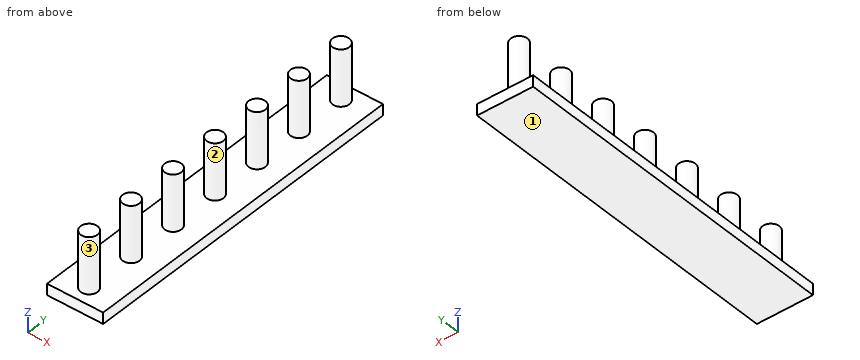
from build123d import *

# Parameters (mm, degrees)
SKETCH_1_W      = 100
SKETCH_1_H      = 600
EXTRUDE_1_DEPTH = 20
SKETCH_2_R      = 15
EXTRUDE_2_DEPTH = 100


with BuildPart() as part:
    # 草图1 → 凸台-拉伸1 (new body)
    with BuildSketch(Plane.XY):
        Rectangle(SKETCH_1_W, SKETCH_1_H)
    extrude(amount=EXTRUDE_1_DEPTH)

    # 草图2 → 凸台-拉伸2 (add)
    with BuildSketch(Plane.XY.offset(20)):
        Circle(SKETCH_2_R)
        with Locations((0, 90)):
            Circle(SKETCH_2_R)
        with Locations((0, 180)):
            Circle(SKETCH_2_R)
        with Locations((0, 270)):
            Circle(SKETCH_2_R)
        with Locations((0, -90)):
            Circle(SKETCH_2_R)
        with Locations((0, -180)):
            Circle(SKETCH_2_R)
        with Locations((0, -270)):
            Circle(SKETCH_2_R)
    extrude(amount=EXTRUDE_2_DEPTH)


solid = part.part
The listing builds one solid part. Answer for the finished solid, in the listing's coordinates (mm). Face numbers are marked on the shaded views. Round coordinates to 2 decimals unless told otherwise and drop trailing zeros. Loops run counter-clockwise (first coordinate to the right, second up) from the corner with the lowest first, then second, coordinate; pieces in that order, holes last. Notation, with made-up numbers: M 24,-5 L 75,-5 A32 cw 75,26 Z; hole C 34.25,61.5 d11. An arc over 180 degrees is marked long. Return JSON: item names as keys, results as strings.
Q1. Find section C-C, the plane y = 180. Determine the outline of the cut face in (x, z).
Results list:
{"outline": "M -50,0 L 50,0 L 50,20 L 15,20 L 15,120 L -15,120 L -15,20 L -50,20 Z"}
Q2. Each of these flat-tipped pins is pushed along its axis until it touches: pin 1 Ø12 at (x, z) = (10, 103.5) entering from +Y; pin 2 Ø10 at (y, z) = (-107, 27.5) entering from +X; pin 3 Ø12 at (x, y) = (21.5, -127) entering from +Z. Where does it stop, or does it pass through?
Results list:
{"pin 1": "stops at y = 284.46", "pin 2": "stops at x = 9", "pin 3": "stops at z = 20"}
Q3. Find the intervals of material crossed by line 1 along Z through (x, y) = (20, 48.5); line 2 along X through (y, z) = (90.5, 66); line 3 along X through (y, z) = (172, 104), in increasing order. Write a range as from..to.
Results list:
{"line 1": "z = 0..20", "line 2": "x = -14.99..14.99", "line 3": "x = -12.69..12.69"}
Q4. Find section A-A, the plane z = 101. Determine the outline of the cut face in (x, y), plus the area to 3 significant figures.
Results list:
{"outline": "C 0,-270 d30; C 0,-180 d30; C 0,-90 d30; C 0,0 d30; C 0,90 d30; C 0,180 d30; C 0,270 d30", "area": "4,950 mm2"}
Q5. Find section D-D, the plane y = 100. Determine the outline of the cut face in (x, z), plus the area to 3 significant figures.
Results list:
{"outline": "M -50,0 L 50,0 L 50,20 L 11.18,20 L 11.18,120 L -11.18,120 L -11.18,20 L -50,20 Z", "area": "4,240 mm2"}
Q6. The mould has two halves that part along Y. Classify the marked faces 1, 2 and 3: released by +Y, released by -Y, zero draft, split by the parting line, or undercut.
Results list:
{"face 1": "zero draft", "face 2": "undercut", "face 3": "undercut"}
